Answer from the drawing. Dimensions are ordinates in mm from the lowest x, y and z of the part. Coordinates: 2 decimals unless noted, no trailing zeros. Write each loop counter-clockwise with the first axis right and the second up, starting at its lowest first coordinate (ties: lowest second). Pieces come first, ordered by that corner, then holes. Notation, with made-up numbers: (46.5, 68.25) - (73.5, 68.25) arc R29 ccw to (73.5, 88.25) - close; hole circle Ø8 at (88.25, 71.5). An arc over 180 degrees is marked (long way). Return JSON: item names as keys, results as strings.
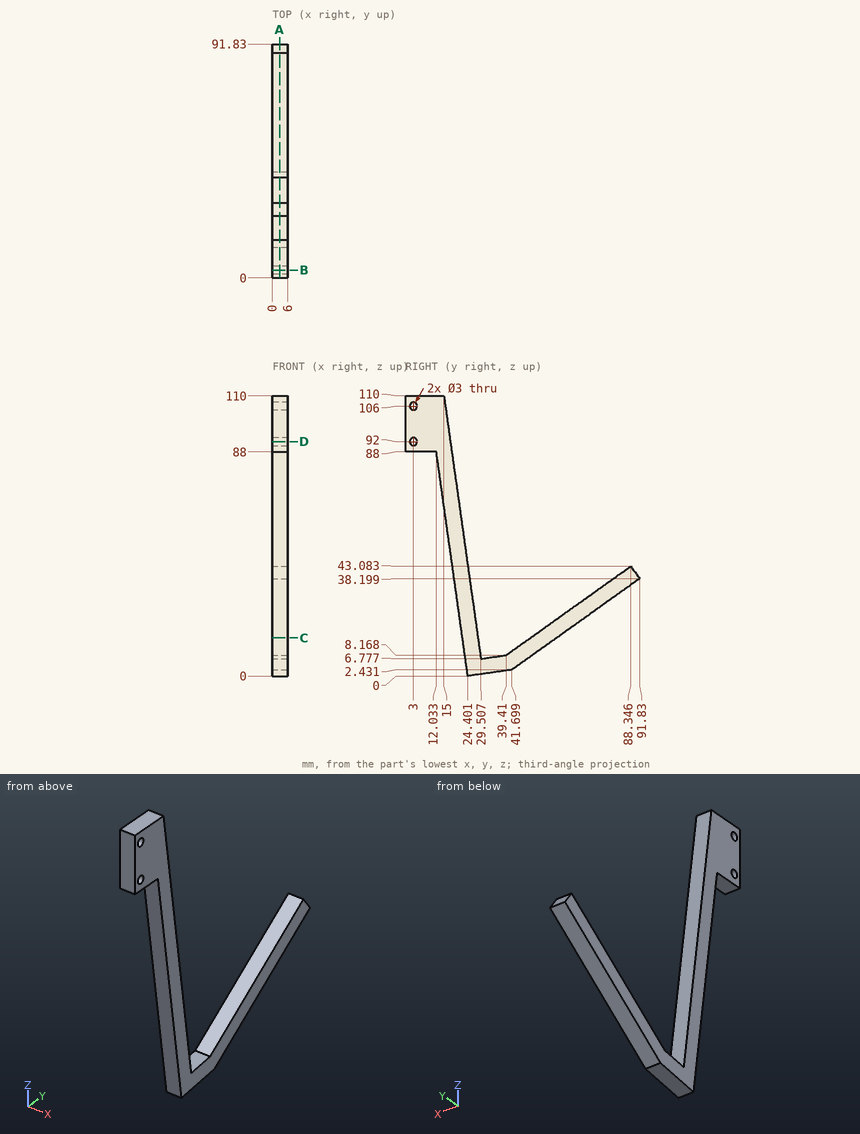
(1) A cutting plane is placed at C-C (z = 15). Determine the outline of the cut face in (x, y) (1 decimal).
Answer:
{"outline": "(0, 22.3) - (6, 22.3) - (6, 28.4) - (0, 28.4) - close; (0, 49) - (6, 49) - (6, 59.3) - (0, 59.3) - close"}
(2) A cutting plane is placed at B-B (y = 3). Determine the outline of the cut face in (x, z).
Answer:
{"outline": "(0, 88) - (6, 88) - (6, 90.5) - (0, 90.5) - close; (0, 93.5) - (6, 93.5) - (6, 104.5) - (0, 104.5) - close; (0, 107.5) - (6, 107.5) - (6, 110) - (0, 110) - close"}
(3) Flat-ended cylindrical pins translate along their axes: P1, Ø1.5, axis at x = 2.5, y = 64.5, coming from the -Z side (1 decimal); P2, Ø3, axis at x = 0.5, y = 62, coming from the +Z side (1 decimal); P3, Ø2, axis at x = 1.5, z = 73, coming from the -Y side. Find the tip coordinate at first contact, or state that the pin passes through.
Answer:
{"P1": "z = 18.2", "P2": "z = 25.4", "P3": "y = 14"}
(4) A cutting plane is placed at D-D (z = 92). Determine the outline of the cut face in (x, y).
Answer:
{"outline": "(0, 0) - (6, 0) - (6, 1.5) - (0, 1.5) - close; (0, 4.5) - (6, 4.5) - (6, 17.53) - (0, 17.53) - close"}
(5) A cutting plane is placed at A-A (x = 2.8). Determine the outline of the cut face in (y, z) (1 decimal), and give its area (3 significant figures).
Answer:
{"outline": "(0, 88) - (12, 88) - (24.4, 0) - (41.7, 2.4) - (91.8, 38.2) - (88.3, 43.1) - (39.4, 8.2) - (29.5, 6.8) - (15, 110) - (0, 110) - close; hole circle Ø3 at (3, 92); hole circle Ø3 at (3, 106)", "area": "1,310 mm²"}
(6) Straight lines are drawn through the part: line 1 (Y direction, x = 1.85, z = 92); line 2 (Y direction, x = 2, z = 13.5) (1 decimal); line 3 (Z direction, x = 4.15, y = 5). For each, find the intervals that lie inside material, in ascending order. Write a range as from..to.
Answer:
{"line 1": "0..1.5, 4.5..17.53", "line 2": "22.5..28.6, 46.9..57.2", "line 3": "88..110"}
